The model under review builds one solid part; all positions refer to its coordinate system, in mm. A direction names the side the tool comes from. Round coordinates to 2 decimals unless told otherwise and drop trailing zeros. Order: outer loops, then holes, each group sorted by start corner. A loop starts at its lowest first (then second) coordinate and runs counter-clockwise, first axis right, second up. Notation, with made-up numbers: M 84,-12.5 L 122,-12.5 A19 ccw 122,22.5 Z; hole C 47,5 d10. An arc over 180 degrees is marked long. Answer as a JSON object with one key per item and string values. Group by question number.
1) Consider section A-A, the plane x = 187. Write out the cut boundary in (y, z).
2) Consider section C-C, the plane y = 0. Write out the cut boundary in (x, z), then the cut area to 3 significant figures.
3) Insertion check: pin 1 Ø5 at (y, z) = (36, -42.5) entering from +X; pin 2 Ø3 at (x, z) = (228.6, -63.5) entering from -Y; pin 3 Ø10 at (y, z) = (17, -26.5) entering from +X; pin 4 Ø1 at (y, z) = (-34, -5) entering from -X. Each pin has a flat end and moves straight along its axis. Give the tip position at first contact, or say it passes through.
4) The part is to be moulded in two halves that separate along X. For faces 3 (the flat face through (232, 44.685, 1)), 4 (the flat face through (225, -48.114, -1)), 5 (the cylindrical face through (505.3, 1.1, 1.1)), 6 (the cylindrical face through (-48.1, -1.1, 1.1)), say which applies: +X half, -X half, draft (parallel to the pull), parting line (faces both ways), or undercut.
5) For faces 1 (the flat face through (225, -44.685, 1)), 2 (the flat face through (230, 47, 76.2)), list the 3-axis set-ups (+Z, -Z, +X, -X, +Y, -Y) from which the entire face can be reached by the end or side of a thin tool; tool diameter is ignored.
6) Consider section B-B, the plane z = 16. Write out the cut boundary in (x, y).
7) To check wall thickness, follow line 1 (Z direction, x = 127, y = -46.35); line 2 (Y direction, x = 134.5, z = 65); line 3 (Z direction, x = 431, y = 46). State the ranges of each line that lie inside material, in increasing order.
```python
from build123d import *

# Parameters (mm, degrees)
SKETCH2_W          = 152.4
SKETCH2_H          = 3.429
SKETCH3_R          = 1.75
CUT_EXTRUDE1_DEPTH = 521.008112247


with BuildPart() as part:
    # Sweep1: sweep along a path in Sketch1
    with BuildLine(Plane.XY) as sweep1_path:
        Line((0, 46.39945), (457.2, 46.39945))
        ThreePointArc((457.2, 46.39945), (503.59945, 0), (457.2, -46.39945))
        Line((457.2, -46.39945), (0, -46.39945))
        ThreePointArc((0, -46.39945), (-46.39945, 0), (0, 46.39945))
    # Sketch2 → Sweep1 (sweep)
    with BuildSketch(Plane(origin=(0, 0, 0), x_dir=(0, 0, -1), z_dir=(1, 0, 0))):
        with Locations((0, 46.39945)):
            Rectangle(SKETCH2_W, SKETCH2_H)
    sweep(path=sweep1_path.line)

    # Sketch3 → Cut-Extrude1 (cut, through all)
    with BuildSketch(Plane(origin=(0, 48.11395, 0), x_dir=(1, 0, 0), z_dir=(0, 1, 0))):
        with Locations(Location((25.4, -63.5, 0), (0, 0, 180))):
            Circle(SKETCH3_R)
        with Locations((25.4, 63.5)):
            Circle(SKETCH3_R)
        with Locations(Location((127, -63.5, 0), (0, 0, 180))):
            Circle(SKETCH3_R)
        with Locations((127, 63.5)):
            Circle(SKETCH3_R)
        with Locations(Location((228.6, -63.5, 0), (0, 0, 180))):
            Circle(SKETCH3_R)
        with Locations((228.6, 63.5)):
            Circle(SKETCH3_R)
        with Locations(Location((330.2, -63.5, 0), (0, 0, 180))):
            Circle(SKETCH3_R)
        with Locations((330.2, 63.5)):
            Circle(SKETCH3_R)
        with Locations(Location((431.8, -63.5, 0), (0, 0, 180))):
            Circle(SKETCH3_R)
        with Locations((431.8, 63.5)):
            Circle(SKETCH3_R)
        with Locations((533.4, -63.5)):
            Circle(SKETCH3_R)
        with Locations((533.4, 63.5)):
            Circle(SKETCH3_R)
    extrude(amount=-CUT_EXTRUDE1_DEPTH, mode=Mode.SUBTRACT)


solid = part.part
```
Results list:
{
 "1": {"outline": "M -48.11,-76.2 L -44.68,-76.2 L -44.68,76.2 L -48.11,76.2 Z; M 44.68,-76.2 L 48.11,-76.2 L 48.11,76.2 L 44.68,76.2 Z"},
 "2": {"outline": "M -48.11,-76.2 L -44.68,-76.2 L -44.68,76.2 L -48.11,76.2 Z; M 501.88,-76.2 L 505.31,-76.2 L 505.31,76.2 L 501.88,76.2 Z", "area": "1,050 mm^2"},
 "3": {"pin 1": "x = 491.74", "pin 2": "through", "pin 3": "x = 503.79", "pin 4": "x = -34.54"},
 "4": {"face 3": "undercut", "face 4": "draft", "face 5": "+X half", "face 6": "-X half"},
 "5": {"face 1": "+Z, -Z", "face 2": "+Z, +X, -X, +Y, -Y"},
 "6": {"outline": "M 0,-48.11 L 457.2,-48.11 A48.11 ccw 457.2,48.11 L 0,48.11 A48.11 ccw Z; hole M 0,-44.68 L 457.2,-44.68 A44.68 ccw 457.2,44.68 L 0,44.68 A44.68 ccw Z"},
 "7": {"line 1": "-76.2 to -65.25, -61.75 to 61.75, 65.25 to 76.2", "line 2": "-48.11 to -44.68, 44.68 to 48.11", "line 3": "-76.2 to -65.06, -61.94 to 61.94, 65.06 to 76.2"}
}
